Here's the drawing with two shaded views (mm, measured from the low corner). I have some questions. Round coordinates to 2 decimals unless told otherwise and drop trailing zeros. Loops run counter-clockwise (first coordinate to the right, second up) from the corner with the lowest first, then second, coordinate; pieces in that order, holes last.
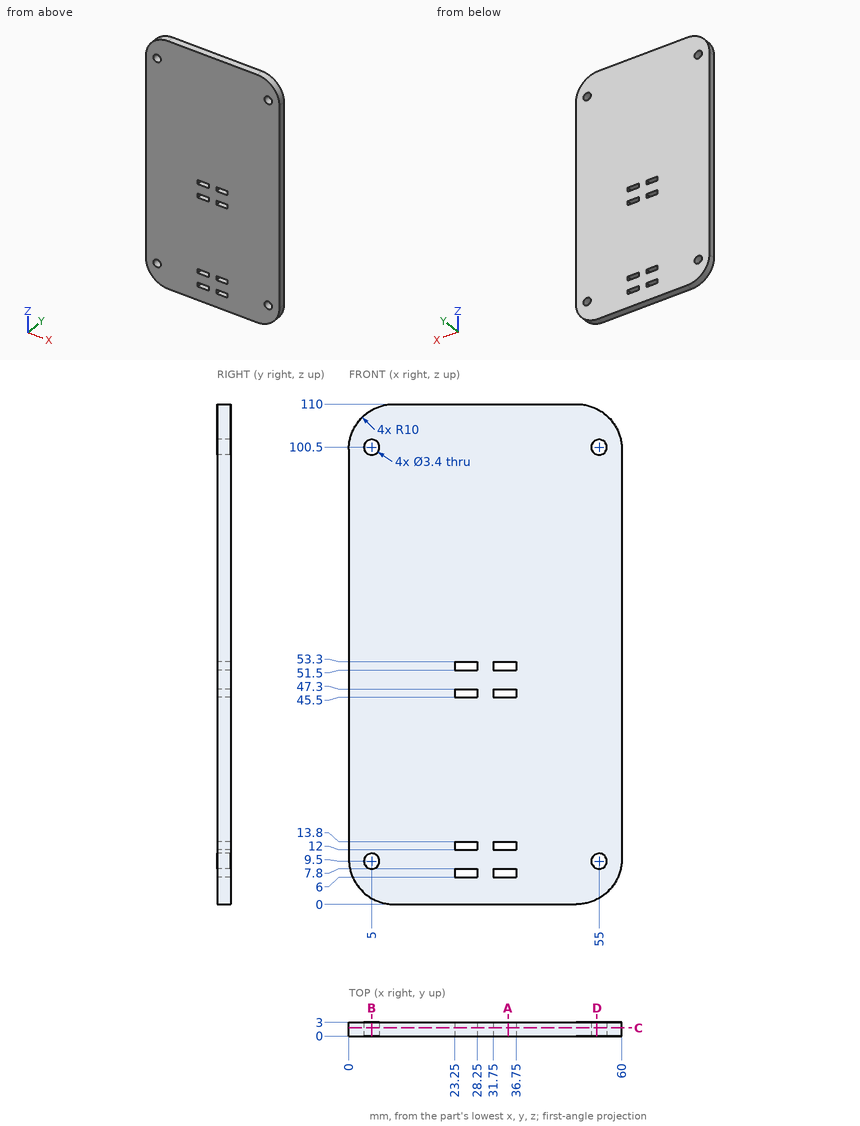
Item 1: If we section it at A-A, the plane x = 35: Please give me the cut outline in (y, z), then the cut area to 3 significant figures.
Results list:
outline: (0, 0) - (3, 0) - (3, 6) - (0, 6) - close; (0, 7.8) - (3, 7.8) - (3, 12) - (0, 12) - close; (0, 13.8) - (3, 13.8) - (3, 45.5) - (0, 45.5) - close; (0, 47.3) - (3, 47.3) - (3, 51.5) - (0, 51.5) - close; (0, 53.3) - (3, 53.3) - (3, 110) - (0, 110) - close
area: 308 mm2
Item 2: Will these pins go through, and if not, where does the flat tip stop? pin 1 (1.4 mm diameter, centred on y = 1, z = 7, fed in from +X); pin 2 (1.4 mm diameter, centred on y = 2, z = 46, fed in from -X); pin 3 (0.5 mm diameter, centred on y = 1.5, z = 7, fed in from -X).
Results list:
pin 1: stops at x = 59.73
pin 2: stops at x = 0
pin 3: stops at x = 0.39
Item 3: If we section it at D-D, the plane x = 54.5: Please give me the cut outline in (y, z), then the cut area to 3 significant figures.
Results list:
outline: (0, 1.07) - (3, 1.07) - (3, 7.88) - (0, 7.88) - close; (0, 11.12) - (3, 11.12) - (3, 98.88) - (0, 98.88) - close; (0, 102.12) - (3, 102.12) - (3, 108.93) - (0, 108.93) - close
area: 304 mm2
Item 4: If I drill on line 1 along X through (y, z) = (2.45, 9.5); line 2 along X through (y, z) = (2.35, 52.5); line 3 along Z through (x, y) = (26, 1.7), over which ranges is the centre line in solid material (lowest first)?
Results list:
line 1: x = 0.01 to 3.3, 6.7 to 53.3, 56.7 to 59.99
line 2: x = 0 to 23.25, 28.25 to 31.75, 36.75 to 60
line 3: z = 0 to 6, 7.8 to 12, 13.8 to 45.5, 47.3 to 51.5, 53.3 to 110
Item 5: If we section it at C-C, the plane y = 1.8: Count the separate pieces of the cut face and the enclosed holes in it, then the cut area to 3 significant figures.
Results list:
separate pieces: 1
enclosed holes: 12
area: 6,410 mm2
Item 6: If we section it at B-B, the plane x = 5: Please give me the cut outline in (y, z), then the cut area to 3 significant figures.
Results list:
outline: (0, 1.34) - (3, 1.34) - (3, 7.8) - (0, 7.8) - close; (0, 11.2) - (3, 11.2) - (3, 98.8) - (0, 98.8) - close; (0, 102.2) - (3, 102.2) - (3, 108.66) - (0, 108.66) - close
area: 302 mm2
